```python
from build123d import *

# Parameters (mm, degrees)
F1_DEPTH = 25.4


with BuildPart() as f1:
    # F0 (on Top) → F1 (new body)
    with BuildSketch(Plane.XY):
        with BuildLine():
            Line((158.613705, 51.07949), (-95.386295, 51.07949))
            ThreePointArc((-95.386295, 51.07949), (-113.217115, 0.27949), (-95.386295, -50.52051))
            Line((-95.386295, -50.52051), (31.613705, -50.52051))
            Line((31.613705, -50.52051), (158.613705, -50.52051))
            ThreePointArc((158.613705, -50.52051), (176.444525, 0.27949), (158.613705, 51.07949))
        make_face()
        with BuildLine():
            Line((145.913705, -37.82051), (31.613705, -37.82051))
            Line((31.613705, -37.82051), (-82.686295, -37.82051))
            ThreePointArc((-82.686295, -37.82051), (-96.05941, 0.27949), (-82.686295, 38.37949))
            Line((-82.686295, 38.37949), (31.613705, 38.37949))
            Line((31.613705, 38.37949), (145.913705, 38.37949))
            ThreePointArc((145.913705, 38.37949), (159.28682, 0.27949), (145.913705, -37.82051))
        make_face(mode=Mode.SUBTRACT)
    extrude(amount=F1_DEPTH)


solid = f1.part
```
Part model, mm, in its own coordinate system. A direction names the side the tool comes from. Coordinates: 2 decimals unless noted, no trailing zeros. Order: outer loops, then holes, each group sorted by start corner. A loop starts at its lowest first (then second) coordinate and runs counter-clockwise, first axis right, second up. Notation, with made-up numbers: (-11.75, 65.25) - (-0.75, 65.25) arc R18 ccw to (-0.75, 70.25) - close; hole circle Ø7 at (39.25, -1). An arc over 180 degrees is marked (long way). Return JSON: item names as keys, results as strings. Group by question number.
Item 1: Pull direction X, two halves, no side cores. Call faces 1 (the face through (-96.057, -0.297, 12.522)), 2 (the face through (33, 51.079, 13)), 3 (the face through (176.44, -0.49, 12.52)), 4 (the face through (30, 38.379, 13)): pulls with the +X half, pulls with the -X half, needs draft (parallel to the pull), parting line crosses it, or undercut.
Item 2: Cut at A-A (x = 101.5). List the corners of the cut face in (y, z).
Item 3: Cut at C-C (y = -34). List the corners of the cut face in (x, z).
Item 4: Cut at B-B (z = 20.75). List the corners of the cut face in (x, y).
Item 5: Which spindle directions (+Z, -Z, +X, -X, +Y, -Y) get a long thin tool onto all of the face, cutting with end or side? Do faces 5 (the face through (159.284, 0.856, 12.522)), 6 (the face through (30, -50.521, 13)). Say none if no direction does.
Item 6: Drill centre lines: probe 1 along Y at (x, z) = (-21, 3.75); probe 2 along X at (y, z) = (-3, 19.25); probe 3 along X at (y, z) = (-11, 9.5). Where is each one in solid material? Low to high. Write a range as from..to.
Check values:
{
 "1": {"face 1": "undercut", "face 2": "needs draft", "face 3": "pulls with the +X half", "face 4": "undercut"},
 "2": {"outline": "(-50.52, 0) - (-37.82, 0) - (-37.82, 25.4) - (-50.52, 25.4) - close; (38.38, 0) - (51.08, 0) - (51.08, 25.4) - (38.38, 25.4) - close"},
 "3": {"outline": "(-105.63, 0) - (-85.51, 0) - (-85.51, 25.4) - (-105.63, 25.4) - close; (148.74, 0) - (168.86, 0) - (168.86, 25.4) - (148.74, 25.4) - close"},
 "4": {"outline": "(-95.39, -50.52) - (158.61, -50.52) arc R81.28 ccw to (158.61, 51.08) - (-95.39, 51.08) arc R81.28 ccw to start; hole (-82.69, -37.82) - (145.91, -37.82) arc R60.96 ccw to (145.91, 38.38) - (-82.69, 38.38) arc R60.96 ccw to start"},
 "5": {"face 5": "+Z, -Z", "face 6": "+Z, -Z, +X, -X, -Y"},
 "6": {"probe 1": "y = -50.52..-37.82, 38.38..51.08", "probe 2": "x = -113.15..-95.97, 159.2..176.38", "probe 3": "x = -112.43..-95.01, 158.23..175.66"}
}
